Part print with two shaded views. Sizes in mm from the minimum x, y, z corner. A direction names the side the tool comes from. Round coordinates to 2 decimals unless told otherwise and drop trailing zeros. Loops run counter-clockwise (first coordinate to the right, second up) from the corner with the lowest first, then second, coordinate; pieces in that order, holes last. Notation, with made-up numbers: (-27, 39) - (25, 39) arc R18 ccw to (25, 68) - close; hole circle Ø3 at (44.5, 85.25). An arc over 180 degrees is marked (long way). Write each question's results on one line, items separated by ' | '. Start each with the question number.
(1) Cut at A-A, the plane x = 54.5. List the corners of the cut face in (y, z), then the cut area to 3 significant figures.
(2) Cut at B-B, the plane z = 54. List the corners of the cut face in (x, y), then the cut area to 3 significant figures.
(3) Drill centre lines: L1, parallel to X at y = 38.5, z = 55; L2, parallel to Z at x = 30.5, y = 63; L3, parallel to Y at x = 54, z = 2. Where is each one in solid material? Low to high.
(4) Cut at C-C, the plane y = 15. List the corners of the cut face in (x, z), then the cut area to 3 significant figures.
(5) Tool access for the marked faces 1 and 2: list every direction of +Z, -Z, +X, -X, +Y, -Y with a clear straight run to the whole face (end or side of a thin tool).
(6) Cut at D-D, the plane z = 96. List the corners of the cut face in (x, y), then the cut area to 3 significant figures.
(7) Flat gauge pin, fed straight in: P1, Ø6, axis at x = 83.5, y = 19.5, coming from the +Z side. Where does the tip first touch, or does it go through?
(8) Mould opens along X. For the marked faces 3, 4 and 5 say: released by +X, released by -X, zero draft, split by the parting line, or undercut.
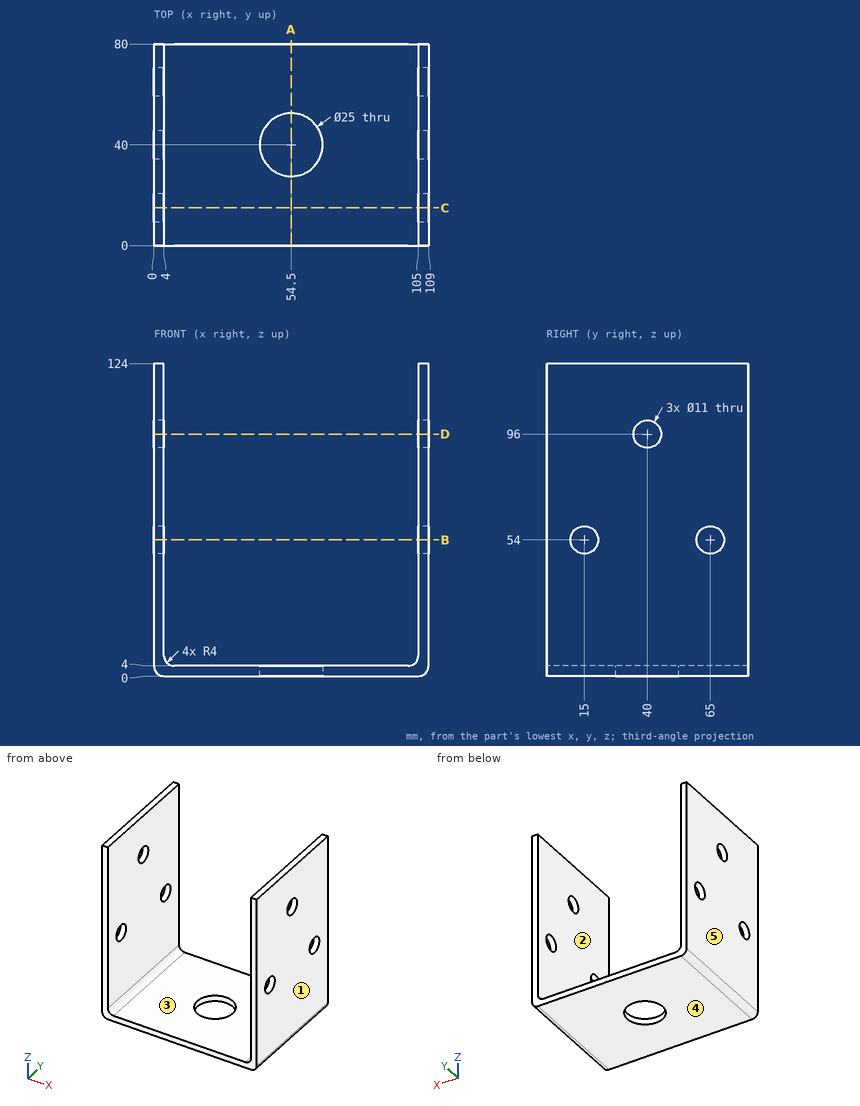
A:
1) outline: (0, 0) - (27.5, 0) - (27.5, 4) - (0, 4) - close; (52.5, 0) - (80, 0) - (80, 4) - (52.5, 4) - close | area: 220 mm2
2) outline: (0, 0) - (4, 0) - (4, 9.5) - (0, 9.5) - close; (0, 20.5) - (4, 20.5) - (4, 59.5) - (0, 59.5) - close; (0, 70.5) - (4, 70.5) - (4, 80) - (0, 80) - close; (105, 0) - (109, 0) - (109, 9.5) - (105, 9.5) - close; (105, 20.5) - (109, 20.5) - (109, 59.5) - (105, 59.5) - close; (105, 70.5) - (109, 70.5) - (109, 80) - (105, 80) - close | area: 464 mm2
3) L1: 0 to 4, 105 to 109 | L2: 0 to 4 | L3: 0 to 27.51, 52.49 to 80
4) outline: (0, 4) arc R4 ccw to (4, 0) - (105, 0) arc R4 ccw to (109, 4) - (109, 48.5) - (105, 48.5) - (105, 8) arc R4 cw to (101, 4) - (8, 4) arc R4 cw to (4, 8) - (4, 48.5) - (0, 48.5) - close; (0, 59.5) - (4, 59.5) - (4, 124) - (0, 124) - close; (105, 59.5) - (109, 59.5) - (109, 124) - (105, 124) - close | area: 1,310 mm2
5) face 1: +Z, -Z, +X, +Y, -Y | face 2: +Z, +Y, -Y
6) outline: (0, 0) - (4, 0) - (4, 34.5) - (0, 34.5) - close; (0, 45.5) - (4, 45.5) - (4, 80) - (0, 80) - close; (105, 0) - (109, 0) - (109, 34.5) - (105, 34.5) - close; (105, 45.5) - (109, 45.5) - (109, 80) - (105, 80) - close | area: 552 mm2
7) P1: z = 4
8) face 3: undercut | face 4: zero draft | face 5: released by -X
